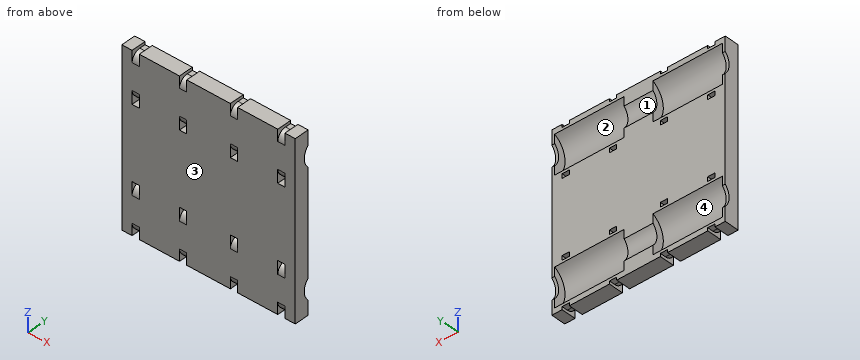
from build123d import *

# Parameters (mm, degrees)
F0_W     = 60
F0_H     = 60
F1_DEPTH = 5
F2_R     = 7.5
F3_DEPTH = 60.001
F4_W     = 1
F4_H     = 60
F4_W_2   = 10
F5_DEPTH = 5
F6_R     = 5
F7_DEPTH = 60.001
F8_W     = 2.5
F8_H     = 1.5
F9_DEPTH = 5.001
F10_R    = 3


with BuildPart() as f1:
    # F0 (on Front) → F1 (new body)
    with BuildSketch(Plane.XZ):
        Rectangle(F0_W, F0_H)
    extrude(amount=F1_DEPTH)

    # F2 (on face) → F3 (cut, through all)
    with BuildSketch(Plane.YZ.offset(30)):
        with Locations((3.5, 21.5)):
            Circle(F2_R)
        with Locations((3.5, -21.5)):
            Circle(F2_R)
    extrude(amount=-F3_DEPTH, mode=Mode.SUBTRACT)

    # F4 (on face) → F5 (join)
    with BuildSketch(Plane(origin=(0, 0, 0), x_dir=(-1, 0, 0), z_dir=(0, 1, 0))):
        with Locations((-29.5, 0)):
            Rectangle(F4_W, F4_H)
        Rectangle(F4_W_2, F4_H)
        with Locations((29.5, 0)):
            Rectangle(F4_W, F4_H)
    extrude(amount=-F5_DEPTH)

    # F6 (on face) → F7 (cut, through all)
    with BuildSketch(Plane.YZ.offset(30)):
        with Locations((3.5, 21.5)):
            Circle(F6_R)
        with Locations((3.5, -21.5)):
            Circle(F6_R)
    extrude(amount=-F7_DEPTH, mode=Mode.SUBTRACT)

    # F8 (on face) → F9 (cut, through all)
    with BuildSketch(Plane(origin=(0, 0, 0), x_dir=(-1, 0, 0), z_dir=(0, 1, 0))):
        with Locations((-25.2, 13.25)):
            Rectangle(F8_W, F8_H)
        with Locations((-8.8, 13.25)):
            Rectangle(F8_W, F8_H)
        with Locations((-8.8, 29.75)):
            Rectangle(F8_W, F8_H)
        with Locations((-25.2, 29.75)):
            Rectangle(F8_W, F8_H)
        with Locations((25.2, 29.75)):
            Rectangle(F8_W, F8_H)
        with Locations((8.8, 13.25)):
            Rectangle(F8_W, F8_H)
        with Locations((8.8, 29.75)):
            Rectangle(F8_W, F8_H)
        with Locations((25.2, 13.25)):
            Rectangle(F8_W, F8_H)
        with Locations((-8.8, -13.25)):
            Rectangle(F8_W, F8_H)
        with Locations((8.8, -29.75)):
            Rectangle(F8_W, F8_H)
        with Locations((25.2, -13.25)):
            Rectangle(F8_W, F8_H)
        with Locations((25.2, -29.75)):
            Rectangle(F8_W, F8_H)
        with Locations((8.8, -13.25)):
            Rectangle(F8_W, F8_H)
        with Locations((-25.2, -13.25)):
            Rectangle(F8_W, F8_H)
        with Locations((-25.2, -29.75)):
            Rectangle(F8_W, F8_H)
        with Locations((-8.8, -29.75)):
            Rectangle(F8_W, F8_H)
    extrude(amount=-F9_DEPTH, mode=Mode.SUBTRACT)

    # F10
    f10_edges = [f1.edges().sort_by_distance(p)[0] for p in [
        (25.2, -5, -29),
        (25.2, -5, -14),
        (8.8, -5, -14),
        (8.8, -5, -29),
        (-8.8, -5, -29),
        (-8.8, -5, -14),
        (-25.2, -5, -14),
        (-25.2, -5, -29),
        (-25.2, -5, 14),
        (-8.8, -5, 14),
        (-8.8, -5, 29),
        (-25.2, -5, 29),
        (8.8, -5, 14),
        (8.8, -5, 29),
        (25.2, -5, 29),
        (25.2, -5, 14),
    ]]
    fillet(f10_edges, radius=F10_R)


solid = f1.part
Verification items for the finished model (mm, model axes). Face numbers are marked on the shaded views. A direction names the side the tool comes from. Give positions to 0.01 mm unless a question says otherwise; leave off trailing zeros. Loops run counter-clockwise (first coordinate to the right, second up) from the corner with the lowest first, then second, coordinate; pieces in that order, holes last.
1) Depth check by flat-ended pin: pin 1 Ø1 at (x, y) = (9, -1) entering from +Z; pin 2 Ø3 at (x, y) = (26, -2) entering from -Z. Enter the tip coordinate at first touch or a pass-through.
2) Draft check along Z on the marked faces 3 and 4. Enter one of: pulls with the +Z half, pulls with the -Z half, needs draft (parallel to the pull), parting line crosses it, or undercut.
3) Sectioned sample at A-A, the plane x = 25. Enter the section's corners in (y, z), then the cut area to 3 significant figures.
4) Sectioned sample at B-B, the plane x = -2. Enter the section's corners in (y, z), then the cut area to 3 significant figures.
5) Sectioned sample at C-C, the plane z = -19. Enter the section's corners in (x, y).
6) Thickness scan on line 1 along X through (y, z) = (-1.2, -26); line 2 along Z through (x, y) = (-1, -0.95); line 3 along Z through (x, y) = (13, -0.5). Record the ranges inside material, lowest first.
7) Set-up check for the marked faces 1 and 2: record each of +Z, -Z, +X, -X, +Y, -Y from which the full face is reachable in a straight line by a thin tool's end or side.
Answers:
1. pin 1: stops at z = 29
1. pin 2: stops at z = -30
2. face 3: needs draft
2. face 4: undercut
3. outline: (-5, -26) arc R3 ccw to (-2, -29) - (0, -29) - (0, -28.13) arc R7.5 cw to (0, -14.87) - (0, -14) - (-2, -14) arc R3 ccw to (-5, -17) - close; (-5, -12.5) - (0, -12.5) - (0, 12.5) - (-5, 12.5) - close; (-5, 17) arc R3 ccw to (-2, 14) - (0, 14) - (0, 14.87) arc R7.5 cw to (0, 28.13) - (0, 29) - (-2, 29) arc R3 ccw to (-5, 26) - close
3. area: 192 mm2
4. outline: (-5, -30) - (0, -30) - (0, -25.07) arc R5 cw to (0, -17.93) - (0, 17.93) arc R5 cw to (0, 25.07) - (0, 30) - (-5, 30) - close
4. area: 285 mm2
5. outline: (-30, -5) - (30, -5) - (30, -0.83) - (29, -0.83) - (29, -3.57) - (5, -3.57) - (5, -0.83) - (-5, -0.83) - (-5, -3.57) - (-29, -3.57) - (-29, -0.83) - (-30, -0.83) - close
6. line 1: x = -30 to -29, -5 to 5, 29 to 30
6. line 2: z = -30 to -23.78, -19.22 to 19.22, 23.78 to 30
6. line 3: z = -30 to -27.84, -15.16 to 15.16, 27.84 to 30
7. face 1: +X, -X, +Y
7. face 2: +Y
